Here's how the part is built. I have some questions about the finished solid (model axes, mm). A direction names the side the tool comes from. Round coordinates to 2 decimals unless told otherwise and drop trailing zeros. Write each loop counter-clockwise with the first axis right and the second up, starting at its lowest first coordinate (ties: lowest second). Pieces come first, ordered by that corner, then holes. Notation, with made-up numbers: (45.5, 18) - (85.5, 18) arc R21 cw to (85.5, 37) - close; hole circle Ø8 at (-6.75, -0.75). An arc over 180 degrees is marked (long way). One line per question, with ' | ' between items. Start each with the question number.
(1) Imagine slicing it at D-D (x = -41). Write out the boundary of the cut face in (y, z), plus the area to 3 significant figures.
(2) If I drill on L1, parallel to Z at x = -16, y = 63; L2, parallel to X at y = -9, z = 17; L3, parallel to Y at x = 45.5, z = 24.5, over which ranges is the centre line in solid material (lowest first)?
(3) Imagine slicing it at C-C (z = 22). Write out the boundary of the cut face in (x, y).
(4) For faces 1 (the flat face through (-1, 1, 0)), 2 (the flat face through (13, 51.366, 23)), 3 (the flat face through (-1, 71.5, 8)), 4 (the flat face through (14, -46.1, 23)), 5 (the flat face through (-37.848, 2, 23)), which set-ups out of +Z, -Z, +X, -X, +Y, -Y let a thin tool reach every point of the face, with its end or its side?
(5) Imagine slicing it at B-B (x = 45.5). Write out the boundary of the cut face in (y, z), plus the area to 3 significant figures.
(6) Will these pins go through, and if not, where does the flat tip stop? pin 1 (4 mm diameter, centred on x = -37, y = -3, fed in from -Z); pin 2 (11 mm diameter, centred on x = 23.5, z = 26, fed in from -Y); pin 3 (5 mm diameter, centred on x = 40, y = 56, fed in from +Z); pin 4 (7 mm diameter, centred on x = -3.5, z = 23, fed in from +Y).
(7) Imagine slicing it at A-A (y = 42.5). Write out the boundary of the cut face in (x, z).
from build123d import *

# Parameters (mm, degrees)
F0_W     = 130
F0_H     = 143
F1_DEPTH = 29.5
F3_DEPTH = 13.5


with BuildPart() as f1:
    # F0 (on Top) → F1 (new body)
    with BuildSketch(Plane.XY):
        Rectangle(F0_W, F0_H)
    extrude(amount=F1_DEPTH)

    # F2 (on face) → F3 (cut)
    with BuildSketch(Plane.XY.offset(29.5)):
        Polygon((-37.84842, 51.365882), (65, 51.365882), (65, 71.5), (-65, 71.5), (-65, -71.5), (65, -71.5), (65, -46.1), (-37.84842, -46.1), align=None)
    extrude(amount=-F3_DEPTH, mode=Mode.SUBTRACT)


solid = f1.part
Check sheet entries:
1) outline: (-71.5, 0) - (71.5, 0) - (71.5, 16) - (-71.5, 16) - close | area: 2,290 mm^2
2) L1: 0 to 16 | L2: -37.85 to 65 | L3: -46.1 to 51.37
3) outline: (-37.85, -46.1) - (65, -46.1) - (65, 51.37) - (-37.85, 51.37) - close
4) face 1: -Z, +X, -X, +Y, -Y | face 2: +Z, +X, -X, +Y | face 3: +Z, -Z, +X, -X, +Y | face 4: +Z, +X, -X, -Y | face 5: +Z, -X, +Y, -Y
5) outline: (-71.5, 0) - (71.5, 0) - (71.5, 16) - (51.37, 16) - (51.37, 29.5) - (-46.1, 29.5) - (-46.1, 16) - (-71.5, 16) - close | area: 3,600 mm^2
6) pin 1: z = 0 | pin 2: y = -46.1 | pin 3: z = 16 | pin 4: y = 51.37
7) outline: (-65, 0) - (65, 0) - (65, 29.5) - (-37.85, 29.5) - (-37.85, 16) - (-65, 16) - close
